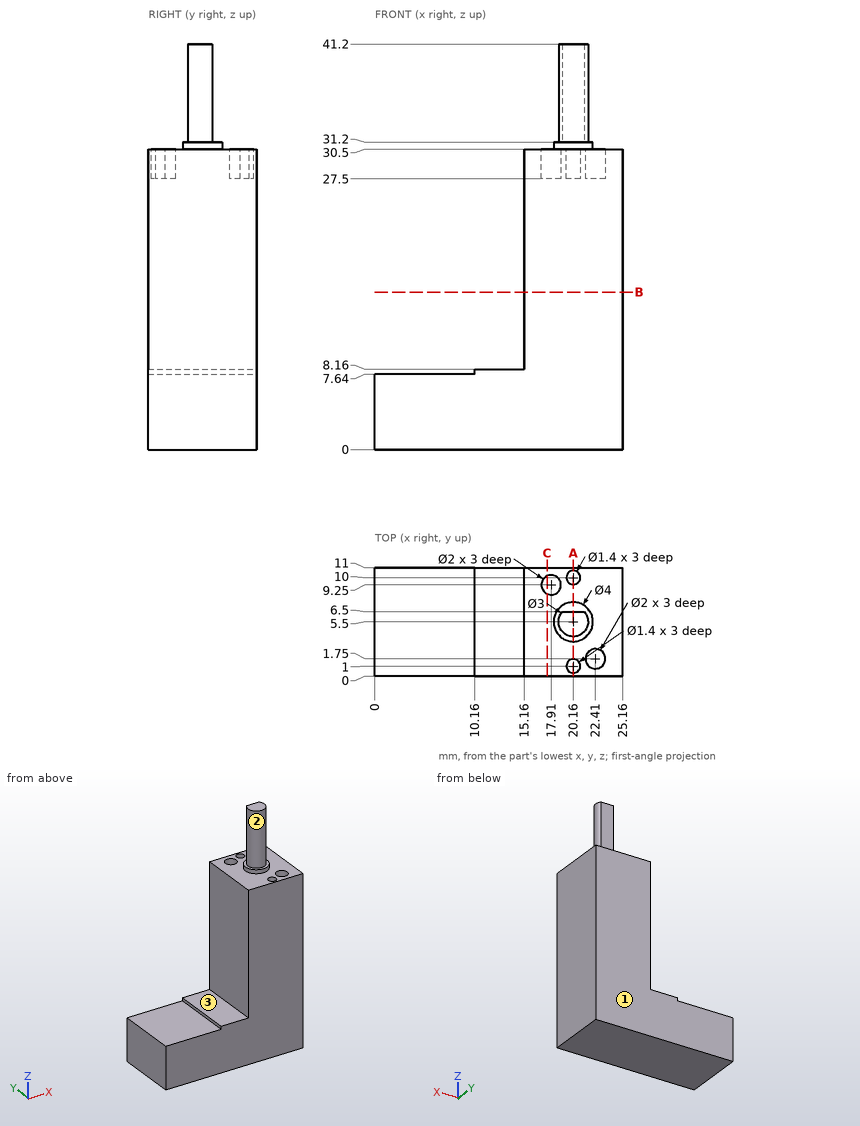
For this review, use the dimensioned drawing (mm, ordinates from the lowest corner) and the shaded views. A direction names the side the tool comes from. Give positions to 0.01 mm unless a question says otherwise; leave off trailing zeros. Order: outer loops, then holes, each group sorted by start corner. A loop starts at its lowest first (then second) coordinate and runs counter-clockwise, first axis right, second up.
1) Take a section at B-B (z = 16). Give the boundary of the cut face in (x, y), then the cut area to 3 significant figures.
2) For the marked faces 1, 2 and 3, list the 3-axis set-ups (+Z, -Z, +X, -X, +Y, -Y) from which the entire face can be reached by the end or side of a thin tool; tool diameter is ignored.
3) Take a section at A-A (x = 20.16). Give the boundary of the cut face in (y, z), then the cut area to 3 significant figures.
4) Insertion check: pin 1 (1.6 mm diameter, centred on x = 17.91, y = 9.25, fed in from +Z); pin 2 (3.5 mm diameter, centred on y = 3.5, z = 19.5, fed in from -X); pin 3 (3 mm diameter, centred on x = 3.5, y = 8, fed in from +Z). Each pin has a flat end and moves straight along its axis. Give the tip position at first contact, or say it passes through.
5) Take a section at C-C (x = 17.5). Give the boundary of the cut face in (y, z), then the cut area to 3 significant figures.
6) Wall thickness on line 1 (Y direction, x = 20.16, z = 29.8); line 2 (Y direction, x = 22.41, z = 29.55); line 3 (Y direction, x = 17.91, z = 29.4): over which ranges is each line inside the solid? List them lowest first.
Derived:
1. outline: (15.16, 0) - (25.16, 0) - (25.16, 11) - (15.16, 11) - close
1. area: 110 mm2
2. face 1: +Z, -Z, +X, -X, +Y
2. face 2: +Z
2. face 3: +Z, -X, +Y, -Y
3. outline: (0, 0) - (11, 0) - (11, 30.5) - (10.7, 30.5) - (10.7, 27.5) - (9.3, 27.5) - (9.3, 30.5) - (7.5, 30.5) - (7.5, 31.2) - (6.5, 31.2) - (6.5, 41.2) - (4, 41.2) - (4, 31.2) - (3.5, 31.2) - (3.5, 30.5) - (1.7, 30.5) - (1.7, 27.5) - (0.3, 27.5) - (0.3, 30.5) - (0, 30.5) - close
3. area: 355 mm2
4. pin 1: stops at z = 27.5
4. pin 2: stops at x = 15.16
4. pin 3: stops at z = 7.64
5. outline: (0, 0) - (11, 0) - (11, 30.5) - (10.16, 30.5) - (10.16, 27.5) - (8.34, 27.5) - (8.34, 30.5) - (0, 30.5) - close
5. area: 330 mm2
6. line 1: y = 0 to 0.3, 1.7 to 9.3, 10.7 to 11
6. line 2: y = 0 to 0.75, 2.75 to 11
6. line 3: y = 0 to 8.25, 10.25 to 11
